from build123d import *

# Parameters (mm, degrees)
SKETCH_1_W          = 67.9
SKETCH_1_H          = 71.85
EXTRUDE_1_DEPTH     = 2
SKETCH_2_W          = 59.9
SKETCH_2_H          = 51.35
EXTRUDE_2_DEPTH     = 1.5
SKETCH_3_W          = 57.9
SKETCH_3_H          = 49.35
EXTRUDE_3_DEPTH     = 14.15
SKETCH_4_R          = 1.8
CUT_EXTRUDE_1_DEPTH = 53.485527767
FILLET_1_R          = 2
FILLET_2_R          = 1.5
FILLET_3_R          = 1
CUT_EXTRUDE_2_DEPTH = 53.485527767
FILLET_4_R          = 2
SKETCH_7_W          = 11
SKETCH_7_H          = 4
EXTRUDE_4_DEPTH     = 1
FILLET_5_R          = 1
SKETCH_8_W          = 8
SKETCH_8_H          = 4
EXTRUDE_5_DEPTH     = 3


with BuildPart() as part:
    # 草图1 → 凸台-拉伸1 (new body)
    with BuildSketch(Plane.XY):
        Rectangle(SKETCH_1_W, SKETCH_1_H)
    extrude(amount=EXTRUDE_1_DEPTH)

    # 草图2 → 凸台-拉伸2 (add)
    with BuildSketch(Plane.XY.offset(2)):
        with Locations((0, -0.75)):
            Rectangle(SKETCH_2_W, SKETCH_2_H)
    extrude(amount=EXTRUDE_2_DEPTH)

    # 草图3 → 凸台-拉伸3 (add)
    with BuildSketch(Plane.XY.offset(3.5)):
        with Locations((0, -0.75)):
            Rectangle(SKETCH_3_W, SKETCH_3_H)
    extrude(amount=EXTRUDE_3_DEPTH)

    # 草图4 → 切除-拉伸1 (cut, through all)
    with BuildSketch(Plane(origin=(0, 0, 0), x_dir=(-1, 0, 0), z_dir=(0, 0, -1))):
        with Locations((24, 31)):
            Circle(SKETCH_4_R)
        with Locations((-24, 31)):
            Circle(SKETCH_4_R)
        with Locations((-24, -31)):
            Circle(SKETCH_4_R)
        with Locations((24, -31)):
            Circle(SKETCH_4_R)
    extrude(amount=-CUT_EXTRUDE_1_DEPTH, mode=Mode.SUBTRACT)

    # 圆角1
    fillet_1_edges = [part.edges().sort_by_distance(p)[0] for p in [
        (33.95, -35.925, 1),
        (-33.95, -35.925, 1),
        (-33.95, 35.925, 1),
        (33.95, 35.925, 1),
    ]]
    fillet(fillet_1_edges, radius=FILLET_1_R)

    # 圆角2
    fillet_2_edges = [part.edges().sort_by_distance(p)[0] for p in [
        (-29.95, 24.925, 2.75),
        (-29.95, -26.425, 2.75),
        (29.95, -26.425, 2.75),
        (29.95, 24.925, 2.75),
    ]]
    fillet(fillet_2_edges, radius=FILLET_2_R)

    # 圆角3
    fillet_3_edges = [part.edges().sort_by_distance(p)[0] for p in [
        (-28.95, 23.925, 10.575),
        (-28.95, -25.425, 10.575),
        (28.95, -25.425, 10.575),
        (28.95, 23.925, 10.575),
    ]]
    fillet(fillet_3_edges, radius=FILLET_3_R)

    # 草图6 → 切除-拉伸2 (cut, through all)
    with BuildSketch(Plane(origin=(0, 0, 0), x_dir=(-1, 0, 0), z_dir=(0, 0, -1))):
        Polygon((-4.45, 33.925), (4.45, 33.925), (4.45, 28.925), (7.45, 28.925), (7.45, 23.925), (-7.45, 23.925), (-7.45, 28.925), (-4.45, 28.925), align=None)
    extrude(amount=-CUT_EXTRUDE_2_DEPTH, mode=Mode.SUBTRACT)

    # 圆角4
    fillet_4_edges = [part.edges().sort_by_distance(p)[0] for p in [
        (4.45, 28.925, 1),
        (-4.45, 28.925, 1),
    ]]
    fillet(fillet_4_edges, radius=FILLET_4_R)

    # 草图7 → 凸台-拉伸4 (add)
    with BuildSketch(Plane.XY.offset(2)):
        with Locations((0, 33.125)):
            Rectangle(SKETCH_7_W, SKETCH_7_H)
    extrude(amount=EXTRUDE_4_DEPTH)

    # 圆角5
    fillet_5_edges = [part.edges().sort_by_distance(p)[0] for p in [
        (-5.5, 35.125, 2.5),
        (-5.5, 31.125, 2.5),
        (5.5, 31.125, 2.5),
        (5.5, 35.125, 2.5),
    ]]
    fillet(fillet_5_edges, radius=FILLET_5_R)

    # 草图8 → 凸台-拉伸5 (add)
    with BuildSketch(Plane.XY.offset(17.65)):
        with Locations((24.95, 15.625)):
            Rectangle(SKETCH_8_W, SKETCH_8_H)
        with Locations((-24.95, -17.125)):
            Rectangle(SKETCH_8_W, SKETCH_8_H)
    extrude(amount=EXTRUDE_5_DEPTH)


solid = part.part
Verification items for the finished model (mm, model axes). A direction names the side the tool comes from. Give positions to 0.01 mm unless a question says otherwise; leave off trailing zeros. Order: outer loops, then holes, each group sorted by start corner. A loop starts at its lowest first (then second) coordinate and runs counter-clockwise, first axis right, second up. Notation, with made-up numbers: M -27,-1 L 25,-1 A29 cw 25,34 Z; hole C -11.75,59.25 d8. An arc over 180 degrees is marked long. Answer as a JSON object with one key per item and string values. Group by question number.
1) Cross-section at C-C (z = 13.5). Enter the section's corners in (x, y) (3 decimals).
2) Depth check by flat-ended pin: pin 1 Ø1.2 at (x, z) = (18, 3) entering from +Y (3 decimals); pin 2 Ø4 at (y, z) = (-2, 3) entering from +X; pin 3 Ø5 at (x, z) = (22.5, 12.5) entering from +Y (3 decimals); pin 4 Ø8 at (x, z) = (3.5, 15) entering from -Y (3 decimals). Enter the tip coordinate at first touch or a pass-through.
3) Mould release check, pull along Y, two halves, no side actions. Record for faces 1 (the face through (-5.051, 29.495, 1.014)), 2 (the face through (-20.95, -17, 19)), 3 (the face through (25, 13.625, 19)): released by +Y, released by -Y, zero draft, split by the parting line, or undercut.
4) Cross-section at D-D (y = 9.5). Enter the section's corners in (x, z), then the cut area to 3 significant figures.
5) Cross-section at A-A (x = 24). Enter the section's corners in (y, z) (3 decimals), then the cut area to 3 significant figures.
6) Access from +Z, -Z, +X, -X, +Y, -Y to the whole of each face (thin tool, end or side, straight path). Record for faces 4 (the face through (7.45, 26, 1)), 5 (the face through (0, -29, 2)), 6 (the face through (-28.95, -1, 10)), 7 (the face through (0, 33, 2)).
7) Scan lines: line 1 along Y through (x, z) = (24, 1.4) (3 decimals); line 2 along X through (y, z) = (10.5, 8). Record each from-to range of solid material in increasing order. Write a range as [from, to].
8) Cross-section at B-B (y = -31). Enter the section's corners in (x, z), then the cut area to 3 significant figures.
Result sheet:
{
 "1": {"outline": "M -28.95,-24.425 A1 ccw -27.95,-25.425 L 27.95,-25.425 A1 ccw 28.95,-24.425 L 28.95,22.925 A1 ccw 27.95,23.925 L -27.95,23.925 A1 ccw -28.95,22.925 Z"},
 "2": {"pin 1": "stops at y = 24.925", "pin 2": "stops at x = 33.95", "pin 3": "stops at y = 23.925", "pin 4": "stops at y = -25.425"},
 "3": {"face 1": "undercut", "face 2": "zero draft", "face 3": "released by -Y"},
 "4": {"outline": "M -33.95,0 L 33.95,0 L 33.95,2 L 29.95,2 L 29.95,3.5 L 28.95,3.5 L 28.95,17.65 L -28.95,17.65 L -28.95,3.5 L -29.95,3.5 L -29.95,2 L -33.95,2 Z", "area": "1,040 mm2"},
 "5": {"outline": "M -35.925,0 L -32.8,0 L -32.8,2 L -35.925,2 Z; M -29.2,0 L 29.2,0 L 29.2,2 L 24.925,2 L 24.925,3.5 L 23.925,3.5 L 23.925,17.65 L 17.625,17.65 L 17.625,20.65 L 13.625,20.65 L 13.625,17.65 L -25.425,17.65 L -25.425,3.5 L -26.425,3.5 L -26.425,2 L -29.2,2 Z; M 32.8,0 L 35.925,0 L 35.925,2 L 32.8,2 Z", "area": "917 mm2"},
 "6": {"face 4": "+Z, -Z", "face 5": "+Z", "face 6": "+Z, -X, +Y, -Y", "face 7": "-Z"},
 "7": {"line 1": "y = [-35.925, -32.8], [-29.2, 29.2], [32.8, 35.925]", "line 2": "x = [-28.95, 28.95]"},
 "8": {"outline": "M -33.95,0 L -25.8,0 L -25.8,2 L -33.95,2 Z; M -22.2,0 L 22.2,0 L 22.2,2 L -22.2,2 Z; M 25.8,0 L 33.95,0 L 33.95,2 L 25.8,2 Z", "area": "121 mm2"}
}
